Verification items for the finished model (mm, model axes). A direction names the side the tool comes from. Coordinates: 2 decimals unless noted, no trailing zeros. Write each loop counter-clockwise with the first axis right and the second up, starting at its lowest first coordinate (ties: lowest second). Pieces come first, ordered by that corner, then holes. Notation, with made-up numbers: (44.25, 54) - (70.25, 54) arc R4 cw to (70.25, 60) - close; hole circle Ø9 at (-19.75, 84). An arc over 180 degrees is marked (long way). Use one line per item in the form item = value. Start each with the question number.
(1) Tool access check on faces 1 (the flat face through (-7, -1.588, 1)), 2 (the flat face through (-15.875, -2, 1)). Record the directions out of +Z, -Z, +X, -X, +Y, -Y that give a thin tool (end or side, any length) a straight path to the whole face; none if there is none.
(2) Mould release check, pull along Z, two halves, no side actions. Record for faces 3 (the flat face through (13, -3.969, 0)), 4 (the flat face through (0, -3, -96.044)), 5 (the flat face through (0, -2, 99.219)), 6 (the flat face through (0, -2, -99.219)): released by +Z, released by -Z, zero draft, split by the parting line, or undercut.
(3) Gauge pin test, flat end, axial feed: pin 1 Ø6 at (x, z) = (6.5, 23) entering from -Y. Record the tip position at first contact, or that the pin passes through.
(4) Material ranges on line 1 (Z direction, x = 4.5, y = -2.15); line 2 (X direction, y = -0.55, z = -65) (3 decimals); line 3 (X direction, y = -3.8, z = -84) (3 decimals), recorded low to high. Write a range as [from, to].
(5) Sectioned sample at A-A (z = -30). Record the cut outline in (x, y) (1 decimal), and give its area (3 significant figures).
(6) Sectioned sample at B-B (y = -0.8). Record the cut outline in (x, z) (3 decimals), and give its area (3 significant figures).
(7) Sectioned sample at C-C (x = 8.5). Record the cut outline in (y, z).
from build123d import *

# Parameters (mm, degrees)
F1_DEPTH = 3.96875
F0_W     = 12.319
F0_H     = 96.04375
F2_DEPTH = 1.5875


with BuildPart() as f1:
    # F0 (on Front) → F1 (new body)
    with BuildSketch(Plane.XZ):
        Polygon((12.7, -96.04375), (15.875, -99.21875), (15.875, 99.21875), (12.7, 96.04375), (12.7, 0), align=None)
        Polygon((-15.875, -99.21875), (-12.7, -96.04375), (-12.7, 0), (-12.7, 96.04375), (-15.875, 99.21875), align=None)
        Polygon((-15.875, 99.21875), (-12.7, 96.04375), (-0.381, 96.04375), (0.381, 96.04375), (12.7, 96.04375), (15.875, 99.21875), align=None)
        Polygon((-0.381, -96.04375), (-12.7, -96.04375), (-15.875, -99.21875), (15.875, -99.21875), (12.7, -96.04375), (0.381, -96.04375), align=None)
    extrude(amount=F1_DEPTH)

    # F0 (on Front) → F2 (join)
    with BuildSketch(Plane.XZ):
        with Locations((6.5405, 48.021875)):
            Rectangle(F0_W, F0_H)
        with Locations((-6.5405, 48.021875)):
            Rectangle(F0_W, F0_H)
        with Locations((-6.5405, -48.021875)):
            Rectangle(F0_W, F0_H)
        with Locations((6.5405, -48.021875)):
            Rectangle(F0_W, F0_H)
    extrude(amount=F2_DEPTH)


solid = f1.part
Answers below:
q1.face_1 = -Y
q1.face_2 = +Z, -Z, -X, +Y, -Y
q2.face_3 = zero draft
q2.face_4 = undercut
q2.face_5 = released by +Z
q2.face_6 = released by -Z
q3.pin_1 = -1.59
q4.line_1 = [-99.22, -96.04], [96.04, 99.22]
q4.line_2 = [-15.875, -0.381], [0.381, 15.875]
q4.line_3 = [-15.875, -12.7], [12.7, 15.875]
q5.outline = (-15.9, -4) - (-12.7, -4) - (-12.7, -1.6) - (-0.4, -1.6) - (-0.4, 0) - (-15.9, 0) - close; (0.4, -1.6) - (12.7, -1.6) - (12.7, -4) - (15.9, -4) - (15.9, 0) - (0.4, 0) - close
q5.area = 64.3 mm2
q6.outline = (-15.875, -99.219) - (15.875, -99.219) - (15.875, 99.219) - (-15.875, 99.219) - close; hole (-0.381, -96.044) - (0.381, -96.044) - (0.381, 96.044) - (-0.381, 96.044) - close
q6.area = 6,150 mm2
q7.outline = (-3.97, -99.22) - (0, -99.22) - (0, 99.22) - (-3.97, 99.22) - (-3.97, 96.04) - (-1.59, 96.04) - (-1.59, -96.04) - (-3.97, -96.04) - close
